Build history of the part. All positions in model axes, mm. Face numbers are marked on the shaded views. Coordinates: 2 decimals unless noted, no trailing zeros. Order: outer loops, then holes, each group sorted by start corner. A loop starts at its lowest first (then second) coordinate and runs counter-clockwise, first axis right, second up. Notation, with made-up numbers: (67, 38) - (117, 38) arc R13 cw to (117, 44) - close; hole circle Ø9 at (43, -26.5). An arc over 180 degrees is marked (long way). Return JSON: item names as keys, results as strings.
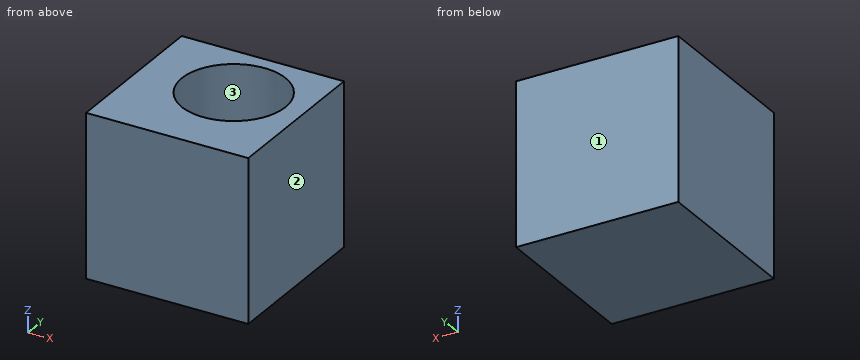
from build123d import *

# Parameters (mm, degrees)
SKETCH101_W      = 5
SKETCH101_H      = 5
EXTRUDE036_DEPTH = 5
SKETCH102_R      = 1.6
HOLE022_DEPTH    = 2.3
HOLE022_TIPS_R   = 1.6


with BuildPart() as part:
    # Sketch101 (on Face9 of Pocket017) → Extrude036 (new body)
    with BuildSketch(Plane.XZ.offset(16.37)):
        with Locations((79.700001, 18.8)):
            Rectangle(SKETCH101_W, SKETCH101_H)
    extrude(amount=EXTRUDE036_DEPTH)

    # Sketch102 (on Face1 of Extrude036) → Hole022 (cut)
    with BuildSketch(Plane.XY.offset(21.3)):
        with Locations((80.000001, -18.4)):
            Circle(SKETCH102_R)
    extrude(amount=-HOLE022_DEPTH, mode=Mode.SUBTRACT)

    # Hole022 tips → Hole022 tip 1 section 0
    with BuildSketch(Plane.XY.offset(19), mode=Mode.PRIVATE) as hole022_tip_1_s0:
        with Locations((80.000001, -18.4)):
            Circle(HOLE022_TIPS_R)
    loft([hole022_tip_1_s0.sketch, Vertex(80.000001, -18.4, 18.038623)], mode=Mode.SUBTRACT)


solid = part.part
1. Cut at A-A on z = 20.15. Give the cut face in (x, y).
Check values:
{"outline": "(77.2, -21.37) - (82.2, -21.37) - (82.2, -16.37) - (77.2, -16.37) - close; hole circle Ø3.2 at (80, -18.4)"}
2. Mould opens along Y. For the marked faces 1, 2 and 3 say: pulls with the +Y half, pulls with the -Y half, needs draft (parallel to the pull), parting line crosses it, or undercut.
Check values:
{"face 1": "pulls with the +Y half", "face 2": "needs draft", "face 3": "undercut"}
3. Drop a flat-ended pin along its axis: pin 1 (2.5 mm diameter, centred on x = 80, y = -18.4, fed in from +Z). Give the stop position or say it passes through.
Check values:
{"pin 1": "z = 18.79"}
4. Probe L1, parallel to Y at x = 80, z = 19.55; L2, parallel to X at y = -17.55, z = 19.05; L3, parallel to Y at x = 80.6, z = 19.5. List the from-to ranges inside material, lowest first.
Check values:
{"L1": "-21.37 to -20, -16.8 to -16.37", "L2": "77.2 to 78.64, 81.36 to 82.2", "L3": "-21.37 to -19.88, -16.92 to -16.37"}
